Input: part model. Units: mm. Frame: model coordinates. A direction names the side the tool comes from. Give positions to 0.01 mm unless a question says otherwise; leave off trailing zeros. Write each loop counter-clockwise with the first axis right and the second up, starting at its lowest first coordinate (ties: lowest second). Pieces come first, ordered by that corner, then holes. Notation, with made-up numbers: (-2, 5) - (15, 5) arc R20 ccw to (15, 20) - close; hole circle Ø6 at (14, 79.5). An arc over 180 degrees is marked (long way). Answer as CSV lines item,"result". Start each with the question number.
from build123d import *

# Parameters (mm, degrees)
SKETCH1_R           = 2.38125
BOSS_EXTRUDE1_DEPTH = 3.175


with BuildPart() as part:
    # Sketch1 → Boss-Extrude1 (new body)
    with BuildSketch(Plane(origin=(0, 0, 0), x_dir=(1, 0, 0), z_dir=(0, 1, 0))):
        with BuildLine():
            Line((-12.7, -38.1), (-12.7, -35.56))
            Line((-12.7, -35.56), (-12.7, 35.56))
            ThreePointArc((-12.7, 35.56), (-11.956051224, 37.356051224), (-10.16, 38.1))
            Line((-10.16, 38.1), (10.16, 38.1))
            ThreePointArc((10.16, 38.1), (11.956051224, 37.356051224), (12.7, 35.56))
            Line((12.7, 35.56), (12.7, -6.35))
            ThreePointArc((12.7, -6.35), (14.559871939, -10.840128061), (19.05, -12.7))
            Line((19.05, -12.7), (69.85, -12.7))
            ThreePointArc((69.85, -12.7), (71.646051224, -13.443948776), (72.39, -15.24))
            Line((72.39, -15.24), (72.39, -35.56))
            ThreePointArc((72.39, -35.56), (71.646051224, -37.356051224), (69.85, -38.1))
            Line((69.85, -38.1), (19.05, -38.1))
            ThreePointArc((19.05, -38.1), (14.559871939, -39.959871939), (12.7, -44.45))
            Line((12.7, -44.45), (12.7, -86.36))
            ThreePointArc((12.7, -86.36), (11.956051224, -88.156051224), (10.16, -88.9))
            Line((10.16, -88.9), (-10.16, -88.9))
            ThreePointArc((-10.16, -88.9), (-11.956051224, -88.156051224), (-12.7, -86.36))
            Line((-12.7, -86.36), (-12.7, -38.1))
        make_face()
        with Locations(Location((0, -25.4, 0), (0, 0, 270))):
            Circle(SKETCH1_R, mode=Mode.SUBTRACT)
        with Locations(Location((0, 0, 0), (0, 0, 270))):
            Circle(SKETCH1_R, mode=Mode.SUBTRACT)
        with Locations(Location((0, 25.4, 0), (0, 0, 270))):
            Circle(SKETCH1_R, mode=Mode.SUBTRACT)
        with Locations(Location((28.575, -25.4, 0), (0, 0, 270))):
            Circle(SKETCH1_R, mode=Mode.SUBTRACT)
        with Locations(Location((57.15, -25.4, 0), (0, 0, 270))):
            Circle(SKETCH1_R, mode=Mode.SUBTRACT)
        with Locations(Location((0, -76.2, 0), (0, 0, 90))):
            Circle(SKETCH1_R, mode=Mode.SUBTRACT)
        with Locations(Location((0, -50.8, 0), (0, 0, 90))):
            Circle(SKETCH1_R, mode=Mode.SUBTRACT)
    extrude(amount=BOSS_EXTRUDE1_DEPTH)


solid = part.part
1) Cut plane C-C on x = 0. Output: boundary loops of the cut face in (y, z) (3 decimals).
2) Cut plane A-A on z = -25.4. Output: boundary loops of the cut face in (x, y) (3 decimals).
3) Cut plane D-D on y = 0.6. State how many separate pieces and enclosed holes the cut face has, and give its area (3 significant figures).
4) Material intervals for line 1 (X direction, y = 2.35, z = 25.4); line 2 (Z direction, x = -1, y = 2.95); line 3 (X direction, y = 1.6, z = 76.2), sorted ascending. Write a range as from..to.
5) Reachability of faces 1 (the flat face through (-12.7, 2, 26)), 2 (the flat face through (12.7, 2, 65)) from +Z, -Z, +X, -X, +Y, -Y: full face, straight path, thin tool, end or side. Return the list, or none.
6) Pull-direction query (Z, two-part tool) for faces 3 (the cylindrical face through (14.61, 1.57, 39.91)), 4 (the cylindrical face through (-0.1, 1.57, 78.58)), 5 (the cylindrical face through (-1.45, 1.57, -1.89)), 6 (the flat face through (72.39, 2, 25)); classes: +Z half, -Z half, draft (parallel to the pull), parting line (faces both ways), or undercut.
7) Cut plane B-B on x = 57.15. Output: boundary loops of the cut face in (y, z) (3 decimals).
8) Contact query for a flat-ended pin moving along its axis: P1, Ø1.6, axis at y = 2, z = 64.5, coming from the +X side. Output: stop coordinate, or through.
Numbers:
1,outline,"(0, -38.1) - (3.175, -38.1) - (3.175, -27.781) - (0, -27.781) - close; (0, -23.019) - (3.175, -23.019) - (3.175, -2.381) - (0, -2.381) - close; (0, 2.381) - (3.175, 2.381) - (3.175, 23.019) - (0, 23.019) - close; (0, 27.781) - (3.175, 27.781) - (3.175, 48.419) - (0, 48.419) - close; (0, 53.181) - (3.175, 53.181) - (3.175, 73.819) - (0, 73.819) - close; (0, 78.581) - (3.175, 78.581) - (3.175, 88.9) - (0, 88.9) - close"
2,outline,"(-12.7, 0) - (-2.381, 0) - (-2.381, 3.175) - (-12.7, 3.175) - close; (2.381, 0) - (12.7, 0) - (12.7, 3.175) - (2.381, 3.175) - close"
3,separate pieces,"1"
3,enclosed holes,"7"
3,area,"4,630 mm²"
4,line 1,"x = -12.7..-2.38, 2.38..26.19, 30.96..54.77, 59.53..72.39"
4,line 2,"z = -38.1..-27.56, -23.24..-2.16, 2.16..23.24, 27.56..48.64, 52.96..74.04, 78.36..88.9"
4,line 3,"x = -12.7..-2.38, 2.38..12.7"
5,face 1,"+Z, -Z, -X, +Y, -Y"
5,face 2,"+Z, +X, +Y, -Y"
6,face 3,"+Z half"
6,face 4,"undercut"
6,face 5,"undercut"
6,face 6,"draft"
7,outline,"(0, 12.7) - (3.175, 12.7) - (3.175, 23.019) - (0, 23.019) - close; (0, 27.781) - (3.175, 27.781) - (3.175, 38.1) - (0, 38.1) - close"
8,P1,"stops at x = 12.7"
